from build123d import *

# Parameters (mm, degrees)
SKETCH1_W                 = 150
SKETCH1_H                 = 400
BOSS_EXTRUDE1_DEPTH       = 18.5
CUT_EXTRUDE1_DEPTH        = 11.5
FILLET1_R                 = 4
CUT_EXTRUDE3_DEPTH        = 8
M6X1_0_TAPPED_HOLE1_D     = 5
M6X1_0_TAPPED_HOLE1_DEPTH = 13.497848452
M6X1_0_TAPPED_HOLE1_TIP   = 1.502151548
CUT_EXTRUDE4_DEPTH        = 11.5
FILLET3_R                 = 4
M5X0_8_TAPPED_HOLE1_D     = 4.2
FILLET5_R                 = 4
CHAMFER2_SIZE             = 1
FILLET6_R                 = 4
CHAMFER3_SIZE             = 3


with BuildPart() as part:
    # Sketch1 → Boss-Extrude1 (new body)
    with BuildSketch(Plane.XY):
        with Locations((61, 100)):
            Rectangle(SKETCH1_W, SKETCH1_H)
    extrude(amount=BOSS_EXTRUDE1_DEPTH)

    # Sketch2 → Cut-Extrude1 (cut)
    with BuildSketch(Plane.XY):
        Polygon((61, 272), (28, 272), (28, 270), (28, 240), (94, 240), (94, 270), (94, 272), align=None)
    extrude(amount=CUT_EXTRUDE1_DEPTH, mode=Mode.SUBTRACT)

    # Fillet1
    fillet1_edges = [part.edges().sort_by_distance(p)[0] for p in [
        (28, 240, 5.75),
        (94, 240, 5.75),
    ]]
    fillet(fillet1_edges, radius=FILLET1_R)

    # Sketch6 → Cut-Extrude3 (cut)
    with BuildSketch(Plane(origin=(0, 0, 0), x_dir=(-1, 0, 0), z_dir=(0, 0, -1))):
        Polygon((-46, 240), (-76, 240), (-79, 240), (-80, 240), (-80, 50), (-80, 44), (-80, -9), (-80, -25), (-42, -25), (-42, -9), (-42, 44), (-42, 50), (-42, 240), (-43, 240), align=None)
    extrude(amount=-CUT_EXTRUDE3_DEPTH, mode=Mode.SUBTRACT)

    # M6x1.0 Tapped Hole1
    with Locations(Plane(origin=(0, 0, 11.5), x_dir=(-1, 0, 0), z_dir=(0, 0, -1))):
        with Locations((-84, 264), (-38, 264), (-38, 251), (-84, 251)):
            Hole(M6X1_0_TAPPED_HOLE1_D / 2, depth=M6X1_0_TAPPED_HOLE1_DEPTH)
            with Locations((0, 0, -(M6X1_0_TAPPED_HOLE1_DEPTH + M6X1_0_TAPPED_HOLE1_TIP / 2))):  # 118° drill point
                Cone(0, M6X1_0_TAPPED_HOLE1_D / 2, M6X1_0_TAPPED_HOLE1_TIP, mode=Mode.SUBTRACT)

    # Sketch11 → Cut-Extrude4 (cut)
    with BuildSketch(Plane(origin=(0, 0, 0), x_dir=(-1, 0, 0), z_dir=(0, 0, -1))):
        with BuildLine():
            Line((-61, 262), (-79, 262))
            Line((-79, 262), (-79, 273))
            ThreePointArc((-79, 273), (-77.828427125, 275.828427125), (-75, 277))
            Line((-75, 277), (-47, 277))
            ThreePointArc((-47, 277), (-44.171572875, 275.828427125), (-43, 273))
            Line((-43, 273), (-43, 262))
            Line((-43, 262), (-61, 262))
        make_face()
    extrude(amount=-CUT_EXTRUDE4_DEPTH, mode=Mode.SUBTRACT)

    # Fillet3
    fillet3_edges = [part.edges().sort_by_distance(p)[0] for p in [
        (28, 272, 5.75),
        (94, 272, 5.75),
        (43, 272, 5.75),
        (79, 272, 5.75),
    ]]
    fillet(fillet3_edges, radius=FILLET3_R)

    # M5x0.8 Tapped Hole1 (through all)
    with Locations(Plane(origin=(0, 0, 0), x_dir=(-1, 0, 0), z_dir=(0, 0, -1))):
        with Locations((-118.5, 280), (-3.5, 280), (-118.5, 220), (-3.5, 220), (-3.5, 160), (-118.5, 160), (-118.5, 100), (-3.5, 100), (-3.5, 40), (-118.5, 40), (-3.5, -20), (-118.5, -20), (-118.5, -80), (-3.5, -80)):
            Hole(M5X0_8_TAPPED_HOLE1_D / 2)

    # Fillet5
    fillet5_edges = [part.edges().sort_by_distance(p)[0] for p in [
        (-14, 300, 9.25),
        (136, 300, 9.25),
        (136, -100, 9.25),
        (-14, -100, 9.25),
    ]]
    fillet(fillet5_edges, radius=FILLET5_R)

    # Chamfer2
    chamfer2_edges = [part.edges().sort_by_distance(p)[0] for p in [
        (1.4, -80, 18.5),
        (116.4, -80, 18.5),
        (116.4, -20, 18.5),
        (1.4, -20, 18.5),
        (116.4, 40, 18.5),
        (1.4, 40, 18.5),
        (1.4, 100, 18.5),
        (116.4, 100, 18.5),
        (116.4, 160, 18.5),
        (1.4, 160, 18.5),
        (1.4, 220, 18.5),
        (116.4, 220, 18.5),
        (1.4, 280, 18.5),
        (116.4, 280, 18.5),
        (61, -100, 18.5),
        (-14, 100, 18.5),
        (136, 100, 18.5),
        (61, 300, 18.5),
        (-12.828427125, 298.828427125, 18.5),
        (134.828427125, 298.828427125, 18.5),
        (134.828427125, -98.828427125, 18.5),
        (-12.828427125, -98.828427125, 18.5),
        (81.5, 251, 18.5),
        (35.5, 251, 18.5),
        (35.5, 264, 18.5),
        (81.5, 264, 18.5),
    ]]
    chamfer(chamfer2_edges, length=CHAMFER2_SIZE)

    # Fillet6
    fillet6_edges = [part.edges().sort_by_distance(p)[0] for p in [
        (42, 240, 4),
        (42, -25, 4),
        (80, -25, 4),
        (80, 240, 4),
    ]]
    fillet(fillet6_edges, radius=FILLET6_R)

    # Chamfer3
    chamfer3_edges = [part.edges().sort_by_distance(p)[0] for p in [
        (61, 277, 0),
        (77.236067977, 276.31662479, 0),
        (44.763932023, 276.31662479, 0),
        (86.208099244, 272, 0),
        (35.791900756, 272, 0),
        (28, 256, 0),
        (80.18013051, 272.68337521, 0),
        (41.81986949, 272.68337521, 0),
        (29.171572875, 270.828427125, 0),
        (92.828427125, 270.828427125, 0),
        (35, 240, 0),
        (94, 256, 0),
        (92.828427125, 241.171572875, 0),
        (29.171572875, 241.171572875, 0),
        (87, 240, 0),
        (42, 107.5, 0),
        (61, -25, 0),
        (80, 107.5, 0),
        (81.171572875, 238.828427125, 0),
        (40.828427125, 238.828427125, 0),
        (43.171572875, -23.828427125, 0),
        (78.828427125, -23.828427125, 0),
    ]]
    chamfer(chamfer3_edges, length=CHAMFER3_SIZE)


solid = part.part
CAD build for the part. Positions are in the model's coordinates, mm. A direction names the side the tool comes from. Coordinates: 2 decimals unless noted, no trailing zeros. Write each loop counter-clockwise with the first axis right and the second up, starting at its lowest first coordinate (ties: lowest second). Pieces come first, ordered by that corner, then holes. Notation, with made-up numbers: (-4.75, -32.5) - (54.25, -32.5) arc R15 ccw to (54.25, -17.5) - close; hole circle Ø10 at (21.5, -21.5). An arc over 180 degrees is marked (long way). Use a Markdown table: item, result. Add a question column.
Item 1: Band-saw the part on A-A, the plane y = 52. Give the cut face in (x, z), and give its area (3 significant figures).
Item 2: Flat gauge pins, fed straight in: pin 1 (6.5 mm diameter, centred on x = 38, y = 264, fed in from +Z); pin 2 (5.5 mm diameter, centred on x = 118.5, y = 40, fed in from +Z); pin 3 (3.5 mm diameter, centred on x = 118.5, y = -20, fed in from -Z); pin 4 (23 mm diameter, centred on x = 57, y = 60.5, fed in from -Z). Where does each tip first touch, or does it go through?
Item 3: Mould opens along X. For faces 3 (the face through (42.32, -24.6, 1.85)), 4 (the face through (27, 103, 0)), 5 (the face through (136, 97, 9)) say: pulls with the +X half, pulls with the -X half, needs draft (parallel to the pull), parting line crosses it, or undercut.
Item 4: Drill centre lines: L1, parallel to X at y = 251, z = 13.55; L2, parallel to Y at x = 84, z = 15.6; L3, parallel to X at y = 62, z = 3.5. Where is each one in solid material? Low to high. Write a range as from..to.
Item 5: 3-axis set-ups, long thin cutter, end or side, ignore diameter. For faces 1 (the face through (61, 259, 11.5)), 2 (the face through (81, 264, 18)): which of +Z, -Z, +X, -X, +Y, -Y reach the whole face in a straight line?
Numbers:
| question | item | result |
|---|---|---|
| 1 | outline | (-14, 0) - (39, 0) - (42, 3) - (42, 8) - (80, 8) - (80, 3) - (83, 0) - (136, 0) - (136, 17.5) - (135, 18.5) - (-13, 18.5) - (-14, 17.5) - close |
| 1 | area | 2,460 mm2 |
| 2 | pin 1 | z = 18.25 |
| 2 | pin 2 | z = 18.15 |
| 2 | pin 3 | through |
| 2 | pin 4 | z = 8 |
| 3 | face 3 | undercut |
| 3 | face 4 | needs draft |
| 3 | face 5 | pulls with the +X half |
| 4 | L1 | -14..35.5, 40.5..81.5, 86.5..136 |
| 4 | L2 | -100..248.5, 253.5..261.5, 266.5..300 |
| 4 | L3 | -14..42, 80..136 |
| 5 | face 1 | -Z |
| 5 | face 2 | +Z |
